Job drawing, mm, ordinate dimensions from the low corner. One solid piece. A direction names the side the tool comes from. Give positions to 0.01 mm unless a question says otherwise; leave off trailing zeros. Write each loop counter-clockwise with the first axis right and the second up, starting at its lowest first coordinate (ties: lowest second). Pieces come first, ordered by that corner, then holes. Notation, with made-up numbers: M 43,26.5 L 69,26.5 A22 cw 69,37.5 Z; hole C -21.5,-19 d1. An arc over 180 degrees is marked long. Use CSV: the item, a comma, the result in double quotes. Start each with the question number.
Item 1: Cut at C-C (z = 5). List the corners of the cut face in (x, y) (3 decimals).
Item 2: Which spindle directions (+Z, -Z, +X, -X, +Y, -Y) get a long thin tool onto all of the face, cutting with end or side? Do the marked faces 4 and 5. Say none if no direction does.
Item 3: Cut at D-D (x = 73.5). List the corners of the cut face in (y, z) (3 decimals).
Item 4: Cut at A-A (x = 50.8). List the corners of the cut face in (y, z) (1 decimal).
Item 5: Mould opens along Y. For the marked faces 1, 2 and 3 say: released by +Y, released by -Y, zero draft, split by the parting line, or undercut.
Item 6: Cut at B-B (y = 8). List the corners of the cut face in (x, z) (3 decimals).
Item 7: Drill centre lines: line 1 (Y direction, x = 83, z = 10.25) (3 decimals); line 2 (Z direction, x = 50.5, y = 20) (3 decimals); line 3 (Z direction, x = 88.9, y = 1.4). Where is each one in solid material? Low to high. Write a range as [from, to].
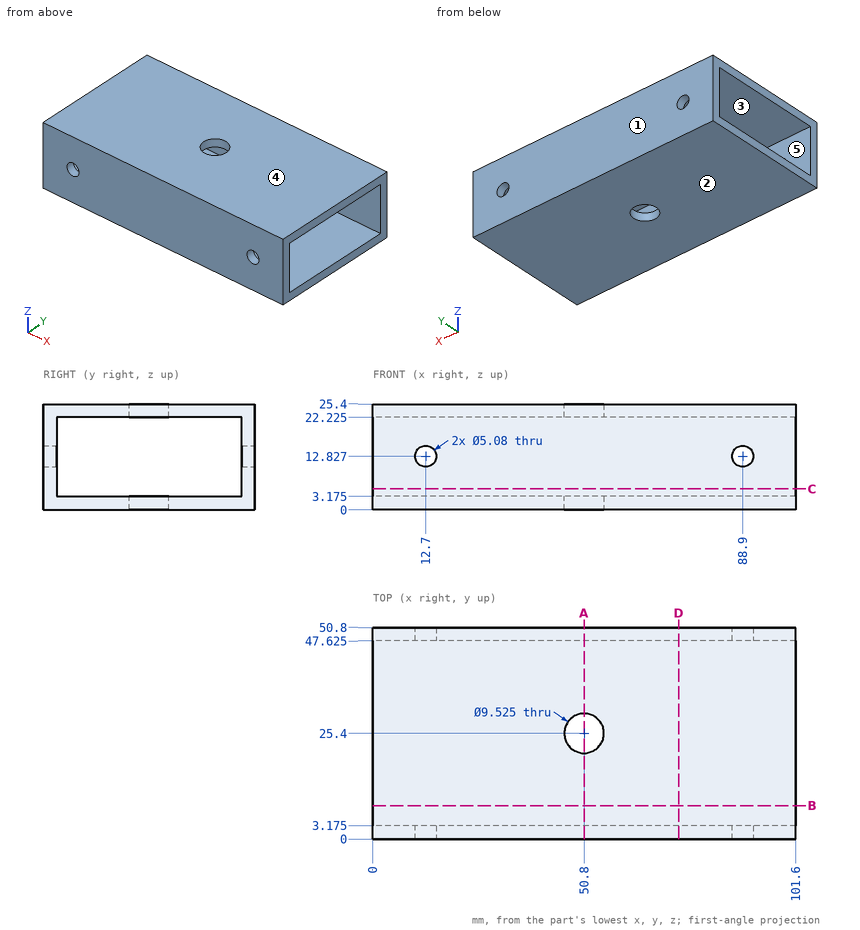
Worked answers:
1,outline,"M 0,0 L 101.6,0 L 101.6,3.175 L 0,3.175 Z; M 0,47.625 L 101.6,47.625 L 101.6,50.8 L 0,50.8 Z"
2,face 4,"+Z, +X, -X, +Y, -Y"
2,face 5,"+X, -X"
3,outline,"M 0,0 L 50.8,0 L 50.8,25.4 L 0,25.4 Z; hole M 3.175,3.175 L 47.625,3.175 L 47.625,22.225 L 3.175,22.225 Z"
4,outline,"M 0,0 L 20.6,0 L 20.6,3.2 L 3.2,3.2 L 3.2,22.2 L 20.6,22.2 L 20.6,25.4 L 0,25.4 Z; M 30.2,0 L 50.8,0 L 50.8,25.4 L 30.2,25.4 L 30.2,22.2 L 47.6,22.2 L 47.6,3.2 L 30.2,3.2 Z"
5,face 1,"released by +Y"
5,face 2,"zero draft"
5,face 3,"undercut"
6,outline,"M 0,0 L 101.6,0 L 101.6,3.175 L 0,3.175 Z; M 0,22.225 L 101.6,22.225 L 101.6,25.4 L 0,25.4 Z"
7,line 1,"y = [0, 3.175], [47.625, 50.8]"
7,line 2,"z = [0, 3.175], [22.225, 25.4]"
7,line 3,"z = [0, 10.29], [15.37, 25.4]"
